Part model, mm, in its own coordinate system. Face numbers are marked on the shaded views. A direction names the side the tool comes from. Give positions to 0.01 mm unless a question says otherwise; leave off trailing zeros. Write each loop counter-clockwise with the first axis right and the second up, starting at its lowest first coordinate (ties: lowest second). Pieces come first, ordered by that corner, then holes.
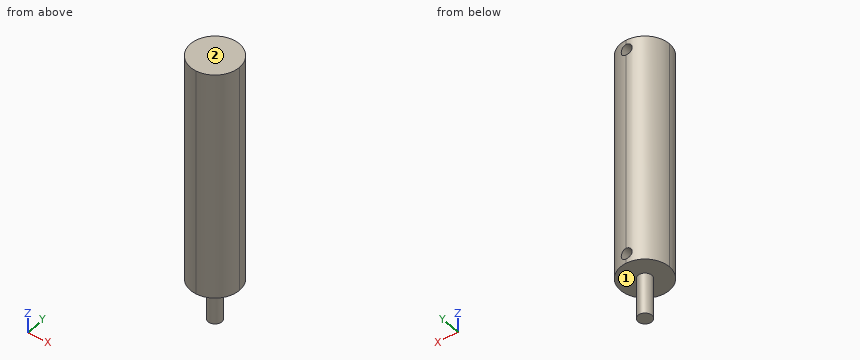
```python
from build123d import *

# Parameters (mm, degrees)
F0_W        = 17.78
F0_H        = 17.78
F1_DEPTH    = 83.82
F2_R        = 2.5
F3_DEPTH    = 15
F4_R        = 2
F5_DEPTH    = 6.35
F6_T1_DEPTH = 128.27


# Not quite as in the source:
# - a fillet or chamfer that OpenCascade refuses, or shapes differently, is made with other operations: its cross-section is extruded or revolved along the edge and cut away or added


with BuildPart() as f1:
    # F0 (on Top) → F1 (new body)
    with BuildSketch(Plane.XY):
        Rectangle(F0_W, F0_H)
    extrude(amount=F1_DEPTH)

    # F2 (on face) → F3 (join)
    with BuildSketch(Plane(origin=(0, 0, 0), x_dir=(1, 0, 0), z_dir=(0, 0, -1))):
        Circle(F2_R)
    extrude(amount=F3_DEPTH)

    # F4 (on face) → F5 (cut)
    with BuildSketch(Plane(origin=(0, 8.89, 0), x_dir=(-1, 0, 0), z_dir=(0, 1, 0))):
        with Locations((0, 3.5875)):
            Circle(F4_R)
        with Locations((0, 80.2325)):
            Circle(F4_R)
    extrude(amount=-F5_DEPTH, mode=Mode.SUBTRACT)

    # F6: fillet of radius 8.89 on 4 edges, made by hand

    # F6_s2 → F6_t1 (cut)
    with BuildSketch(Plane.XY.offset(-22.225)):
        with BuildLine():
            ThreePointArc((8.89, 0), (6.2861792847, -6.2861792847), (0, -8.89))
            Line((0, -8.89), (8.89, -8.89))
            Line((8.89, -8.89), (8.89, 0))
        make_face()
        with BuildLine():
            ThreePointArc((8.89, 0), (6.2861792847, 6.2861792847), (0, 8.89))
            Line((0, 8.89), (8.89, 8.89))
            Line((8.89, 8.89), (8.89, 0))
        make_face()
        with BuildLine():
            ThreePointArc((0, 8.89), (-6.2861792847, 6.2861792847), (-8.89, 0))
            Line((-8.89, 0), (-8.89, 8.89))
            Line((-8.89, 8.89), (0, 8.89))
        make_face()
        with BuildLine():
            ThreePointArc((0, -8.89), (-6.2861792847, -6.2861792847), (-8.89, 0))
            Line((-8.89, 0), (-8.89, -8.89))
            Line((-8.89, -8.89), (0, -8.89))
        make_face()
    extrude(amount=F6_T1_DEPTH, mode=Mode.SUBTRACT)


solid = f1.part
```
1) Saw through at A-A, the plane z = 9. Write the cut outline in (x, y), then the cut area to 3 significant figures.
Answers follow:
outline: circle Ø17.78 at (0, 0)
area: 248 mm2
2) Saw through at B-B, the plane y = 7.5. Write the cut outline in (x, z), then the cut area to 3 significant figures.
Answers follow:
outline: (-4.77, 0) - (4.77, 0) - (4.77, 83.82) - (-4.77, 83.82) - close; hole circle Ø4 at (0, 3.59); hole circle Ø4 at (0, 80.23)
area: 775 mm2
3) Wall check: L1, parallel to Z at x = 0, y = 6; L2, parallel to Z at x = 5.75, y = 0.75; L3, parallel to X at y = -0.25, z = 51. Give the ranges that are in metal, low to high.
Answers follow:
L1: z = 0 to 1.59, 5.59 to 78.23, 82.23 to 83.82
L2: z = 0 to 83.82
L3: x = -8.89 to 8.89
4) Pin check, flat tips, straight feed: pin 1 Ø5 at (x, z) = (0, 80.23) entering from +Y; pin 2 Ø6 at (x, z) = (5, 35) entering from -Y; pin 3 Ø1 at (x, z) = (-2, 0) entering from +Y; pin 4 Ø1.2 at (x, z) = (-1, 4.5) entering from +Y. Stop position of each tip, or through.
Answers follow:
pin 1: stops at y = 8.89
pin 2: stops at y = -8.66
pin 3: stops at y = 8.76
pin 4: stops at y = 2.54
5) Saw through at C-C, the plane x = -5.75. Write the cut outline in (y, z).
Answers follow:
outline: (-6.78, 0) - (6.78, 0) - (6.78, 83.82) - (-6.78, 83.82) - close
6) 3-axis set-ups, long thin cutter, end or side, ignore diameter. For the marked faces 1 and 2: which of +Z, -Z, +X, -X, +Y, -Y reach the whole face in a straight line?
Answers follow:
face 1: -Z
face 2: +Z, +X, -X, +Y, -Y
